Job drawing, mm, ordinate dimensions from the low corner. One solid piece. A direction names the side the tool comes from. Round coordinates to 2 decimals unless told otherwise and drop trailing zeros. Write each loop counter-clockwise with the first axis right and the second up, starting at its lowest first coordinate (ties: lowest second). Pieces come first, ordered by that corner, then holes.
1) Which spindle directions (+Z, -Z, +X, -X, +Y, -Y) get a long thin tool onto all of the face, cutting with end or side? Do the marked faces 1 and 2. Say none if no direction does.
2) Saw through at D-D (y = 6). Write the cut outline in (x, z) (1 decimal), plus the area to 3 significant figures.
3) Pull direction Z, two halves, no side cores. Call the marked faces 3, 4 and 5: +Z half, -Z half, draft (parallel to the pull), parting line (faces both ways), or undercut.
4) Saw through at A-A (z = 15.5). Write the cut outline in (x, y) (1 decimal), plus the area to 3 significant figures.
5) Saw through at C-C (y = 14.5). Write the cut outline in (x, z) (1 decimal), plus the area to 3 significant figures.
6) Flat gauge pins, fed straight in: pin 1 (6 mm diameter, centred on y = 17.5, z = 19.5, fed in from +X); pin 2 (1.5 mm diameter, centred on x = 23, y = 22, fed in from -Z); pin 3 (7 mm diameter, centred on x = 17.95, y = 15.96, fed in from +Z); pin 4 (3 mm diameter, centred on x = 26, y = 18, fed in from +Z). Where does each tip first touch, or does it go through?
7) Saw through at B-B (x = 14.5). Write the cut outline in (y, z).
8) Wall check: probe 1 along Y at (x, z) = (6.5, 18.5) (1 decimal); probe 2 along Z at (x, y) = (13, 14.5). Give the ranges that are in metal, low to high.
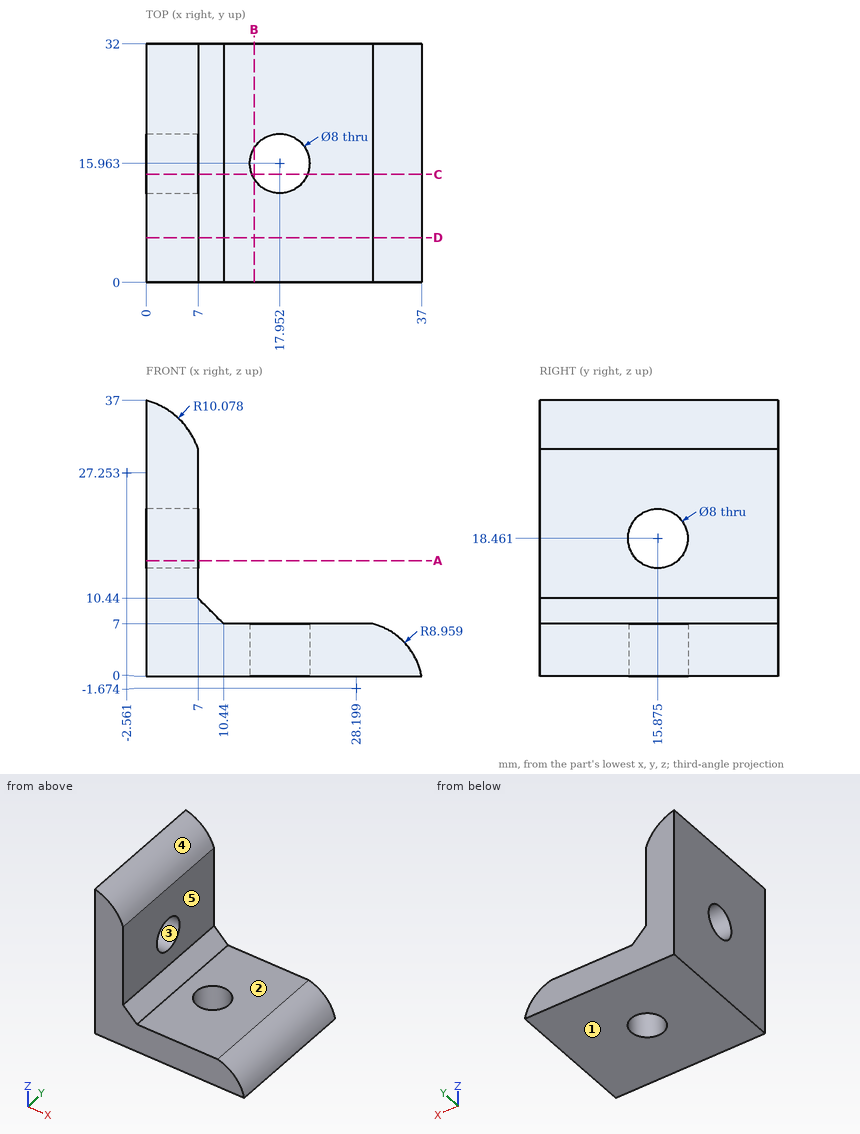
Evaluation:
1. face 1: -Z, +X, -X, +Y, -Y
1. face 2: +Z, +X, +Y, -Y
2. outline: (0, 0) - (37, 0) arc R9 ccw to (30.4, 7) - (10.4, 7) - (7, 10.4) - (7, 30.4) arc R10.1 ccw to (0, 37) - close
2. area: 446 mm2
3. face 3: undercut
3. face 4: +Z half
3. face 5: draft
4. outline: (0, 0) - (7, 0) - (7, 13.2) - (0, 13.2) - close; (0, 18.6) - (7, 18.6) - (7, 32) - (0, 32) - close
4. area: 186 mm2
5. outline: (0, 0) - (14.2, 0) - (14.2, 7) - (10.4, 7) - (7, 10.4) - (7, 14.7) - (0, 14.7) - close; (0, 22.2) - (7, 22.2) - (7, 30.4) arc R10.1 ccw to (0, 37) - close; (21.7, 0) - (37, 0) arc R9 ccw to (30.4, 7) - (21.7, 7) - close
5. area: 341 mm2
6. pin 1: stops at x = 7
6. pin 2: stops at z = 0
6. pin 3: passes through
6. pin 4: stops at z = 7
7. outline: (0, 0) - (13.94, 0) - (13.94, 7) - (0, 7) - close; (17.98, 0) - (32, 0) - (32, 7) - (17.98, 7) - close
8. probe 1: y = 0 to 11.9, 19.9 to 32
8. probe 2: z = 0 to 7
